Source: CAD feature listing. Evaluate the final solid. Frame: model axes, mm. Face numbers are marked on the shaded views. A direction names the side the tool comes from. Give positions to 0.01 mm unless a question says otherwise; leave off trailing zeros. Loops run counter-clockwise (first coordinate to the right, second up) from the corner with the lowest first, then second, coordinate; pieces in that order, holes last. Notation, with made-up numbers: M 50,54.25 L 82,54.25 A29 cw 82,76.25 Z; hole C -10.5,72 d9. An arc over 180 degrees is marked long. Write item = value, one per line.
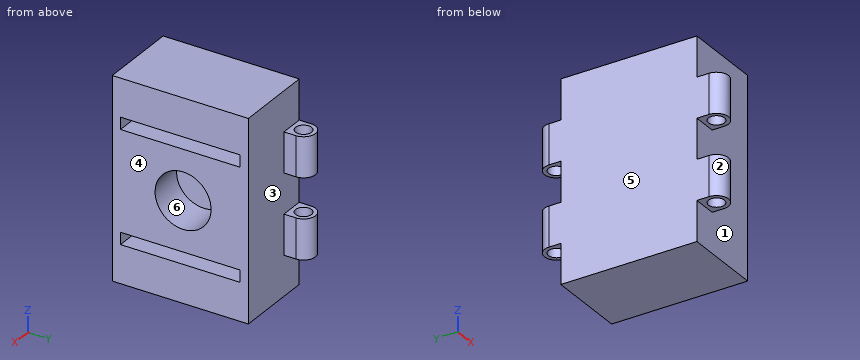
from build123d import *

# Parameters (mm, degrees)
SKETCH1_W                      = 50
SKETCH1_H                      = 34.11
BOSS_EXTRUDE1_DEPTH            = 20
SKETCH3_R                      = 2
BOSS_EXTRUDE2_DEPTH            = 10
LPATTERN1_COUNT                = 2
LPATTERN1_PITCH                = 20
MIRROR1_COPY_1_SKETCH_R        = 2
MIRROR1_COPY_1_DEPTH           = 10
SKETCH5_R                      = 7
CUT_EXTRUDE1_DEPTH             = 10
CUT_EXTRUDE1_DIRECTION_2_REACH = 3.559
SKETCH6_W                      = 3
SKETCH6_H                      = 30
CUT_EXTRUDE2_DEPTH             = 10


with BuildPart() as part:
    # Sketch1 → Boss-Extrude1 (new body)
    with BuildSketch(Plane(origin=(0, 0, 0), x_dir=(0, 0, -1), z_dir=(1, 0, 0))):
        with Locations((25, 17.055)):
            Rectangle(SKETCH1_W, SKETCH1_H)
    extrude(amount=BOSS_EXTRUDE1_DEPTH)

    # Sketch3 → Boss-Extrude2 (add)
    with BuildSketch(Plane.XY.offset(-10)):
        with BuildLine():
            Line((0, 34.11), (0, 37.11))
            ThreePointArc((0, 37.11), (3, 40.11), (6, 37.11))
            Line((6, 37.11), (6, 34.11))
            Line((6, 34.11), (3, 34.11))
            Line((3, 34.11), (0, 34.11))
        make_face()
        with Locations((3, 37.11)):
            Circle(SKETCH3_R, mode=Mode.SUBTRACT)
    boss_extrude2 = extrude(amount=-BOSS_EXTRUDE2_DEPTH)

    # LPattern1: Boss-Extrude2 ×2
    with Locations(*[(0, 0, -i * LPATTERN1_PITCH) for i in range(1, LPATTERN1_COUNT)]):
        add(boss_extrude2)

    # Mirror1: Boss-Extrude2 across plane
    add(boss_extrude2.mirror(Plane.ZX.offset(17.055)))

    # Mirror1 copy 1 sketch → Mirror1 copy 1 (add)
    with BuildSketch(Plane(origin=(0, 34.11, -30), x_dir=(1, 0, 0), z_dir=(0, 0, 1))):
        with BuildLine():
            Line((0, -34.11), (0, -37.11))
            ThreePointArc((0, -37.11), (3, -40.11), (6, -37.11))
            Line((6, -37.11), (6, -34.11))
            Line((6, -34.11), (3, -34.11))
            Line((3, -34.11), (0, -34.11))
        make_face()
        with Locations((3, -37.11)):
            Circle(MIRROR1_COPY_1_SKETCH_R, mode=Mode.SUBTRACT)
    extrude(amount=-MIRROR1_COPY_1_DEPTH)

    # Sketch5 → Cut-Extrude1 (cut)
    with BuildSketch(Plane(origin=(20, 17.754268119, -25), x_dir=(0, 0, -1), z_dir=(0.99756405, 0.069756474, 0))):
        Circle(SKETCH5_R)
    extrude(amount=-CUT_EXTRUDE1_DEPTH, mode=Mode.SUBTRACT)

    # Sketch5 → Cut-Extrude1 direction 2 (cut, up to next)
    with BuildSketch(Plane(origin=(20, 17.754268119, -25), x_dir=(0, 0, -1), z_dir=(0.99756405, 0.069756474, 0)), mode=Mode.PRIVATE) as cut_extrude1_direction_2_sk1:
        Circle(SKETCH5_R)
    cut_extrude1_direction_2_tool1 = extrude(cut_extrude1_direction_2_sk1.sketch, amount=CUT_EXTRUDE1_DIRECTION_2_REACH, mode=Mode.PRIVATE) & part.part
    add(cut_extrude1_direction_2_tool1.solids().sort_by_distance((20, 17.754268, -25))[0], mode=Mode.SUBTRACT)

    # Sketch6 → Cut-Extrude2 (cut)
    with BuildSketch(Plane(origin=(20, 0, 0), x_dir=(0, 0, -1), z_dir=(1, 0, 0))):
        with Locations((11, 17.055)):
            Rectangle(SKETCH6_W, SKETCH6_H)
        with Locations((39, 17.055)):
            Rectangle(SKETCH6_W, SKETCH6_H)
    extrude(amount=-CUT_EXTRUDE2_DEPTH, mode=Mode.SUBTRACT)


solid = part.part
1. Reachability of the marked faces 1, 2 and 3 from +Z, -Z, +X, -X, +Y, -Y: full face, straight path, thin tool, end or side. Return the list, or none.
Derived:
face_1 = +X, -Y
face_2 = +Z, -Z, -Y
face_3 = +X, +Y
2. Cut plane A-A, the plane z = -34. Return the cut outline in (x, y).
Derived:
outline = M 0,-3 A3 ccw 6,-3 L 6,0 L 20,0 L 20,34.11 L 6,34.11 L 6,37.11 A3 ccw 0,37.11 Z; hole C 3,-3 d4; hole C 3,37.11 d4
3. Material intervals for probe 1 along Z at (x, y) = (15.5, 3); probe 2 along Y at (x, z) = (3, -14.5); probe 3 along X at (y, z) = (37, -13), sorted ascending. Write a range as from..to.
Derived:
probe_1 = -50..-40.5, -37.5..-12.5, -9.5..0
probe_2 = -6..-5, -1..35.11, 39.11..40.11
probe_3 = 0..1, 5..6
4. First-contact query: pin 1 Ø6 at (x, z) = (14.5, -13) entering from +Y; pin 2 Ø1.8 at (x, y) = (4, -4) entering from +Z; pin 3 Ø0.9 at (y, z) = (36.5, -35.5) entering from +X. Flat tips, straight axial feed; report the tip coordinate or a pass-through.
Derived:
pin_1 = 34.11
pin_2 = -10
pin_3 = 6
5. Pull-direction query (X, two-part tool) for the marked faces 4, 5 and 6; classes: +X half, -X half, draft (parallel to the pull), parting line (faces both ways), or undercut.
Derived:
face_4 = +X half
face_5 = -X half
face_6 = undercut
6. Cut plane B-B, the plane y = 36. Return the cut outline in (x, z).
Derived:
outline = M 0,-40 L 1.34,-40 L 1.34,-30 L 0,-30 Z; M 0,-20 L 1.34,-20 L 1.34,-10 L 0,-10 Z; M 4.66,-40 L 6,-40 L 6,-30 L 4.66,-30 Z; M 4.66,-20 L 6,-20 L 6,-10 L 4.66,-10 Z
7. Cut plane D-D, the plane x = 8.25. Return the cut outline in (y, z).
Derived:
outline = M 0,-50 L 34.11,-50 L 34.11,0 L 0,0 Z
8. Cut plane C-C, the plane x = 3. Count the separate pieces of the cut face and the enclosed holes in it, then the cut area to 3 significant figures.
Derived:
separate_pieces = 5
enclosed_holes = 0
area = 1,790 mm²
